CAD build for the part. Positions are in the model's coordinates, mm. Face numbers are marked on the shaded views. A direction names the side the tool comes from. Give positions to 0.01 mm unless a question says otherwise; leave off trailing zeros. Write each loop counter-clockwise with the first axis right and the second up, starting at its lowest first coordinate (ties: lowest second). Pieces come first, ordered by that corner, then holes. Notation, with made-up numbers: (14, 62.5) - (44, 62.5) arc R11 cw to (44, 69.5) - close; hole circle Ø4 at (-14, 12). An arc over 180 degrees is marked (long way). Put each result on its own line as item: value. Start each with the question number.
1. Cut at C-C on y = 10.25. List the corners of the cut face in (x, z).
2. Wall check: line 1 (X direction, y = 7.25, z = 0); line 2 (Z direction, x = 1, y = 11.5); line 3 (Z direction, x = -5.75, y = -1.5). Give the ranges that are in metal, low to high.
3. Cut at B-B on y = -0.5. List the corners of the cut face in (x, z).
4. Tool access for the marked faces 1, 2 and 3: list every direction of +Z, -Z, +X, -X, +Y, -Y with a clear straight run to the whole face (end or side of a thin tool).
5. Drop flat-ended pins along their axis: pin 1 (5 mm diameter, centred on x = 7, y = -3, fed in from +Z); pin 2 (3 mm diameter, centred on y = -0.5, z = -7.5, fed in from +X); pin 3 (1.5 mm diameter, centred on x = -3.5, y = -2.5, fed in from -Z); pin 4 (5 mm diameter, centred on x = 4.5, z = -6, fed in from +Y). Give the stop position or say it passes through.
6. Mould opens along Z. For the marked faces 4, 5 and 6 say: +Z half, -Z half, draft (parallel to the pull), parting line (faces both ways), or undercut.
7. Cut at A-A on y = 6. List the corners of the cut face in (x, z).
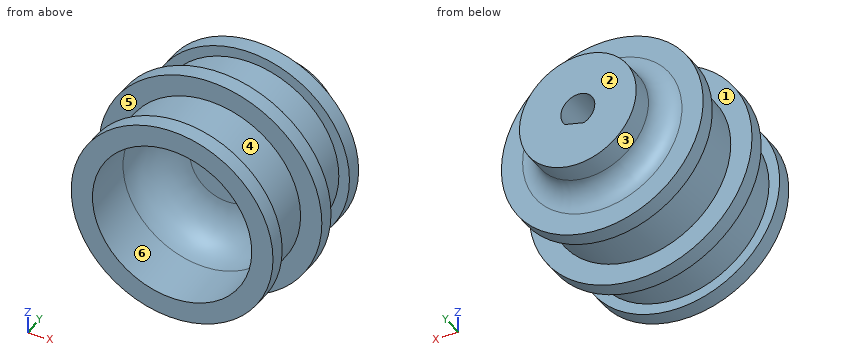
from build123d import *

# Parameters (mm, degrees)
ZAOKR_GLENIE1_R            = 2
WYTNIJ_WYCI_GNI_CIE1_DEPTH = 19


with BuildPart() as part:
    # Szkic1 → Obrót1 (revolve)
    with BuildSketch(Plane.XY):
        with BuildLine():
            Line((7.5, -4.799176992), (7.5, 0.200823008))
            ThreePointArc((7.5, 0.200823008), (6.328427125, 3.029250132), (3.5, 4.200823008))
            Line((3.5, 4.200823008), (0, 4.200823008))
            Line((0, 4.200823008), (0, 13.200823008))
            Line((0, 13.200823008), (5.5, 13.200823008))
            Line((5.5, 13.200823008), (5.5, 9.200823008))
            Line((5.5, 9.200823008), (9.5, 9.200823008))
            Line((9.5, 9.200823008), (9.5, 7.700823008))
            Line((9.5, 7.700823008), (8.5, 7.700823008))
            Line((8.5, 7.700823008), (8.5, 2.950823008))
            Line((8.5, 2.950823008), (10.5, 2.950823008))
            Line((10.5, 2.950823008), (10.5, 1.450823008))
            Line((10.5, 1.450823008), (8.5, 1.450823008))
            Line((8.5, 1.450823008), (8.5, -3.299176992))
            Line((8.5, -3.299176992), (9.5, -3.299176992))
            Line((9.5, -3.299176992), (9.5, -4.799176992))
            Line((9.5, -4.799176992), (7.5, -4.799176992))
        make_face()
    revolve(axis=Axis((0, -15.783107462, 0), (0, 1, 0)))

    # Zaokrąglenie1
    zaokr_glenie1_edges = [part.edges().sort_by_distance(p)[0] for p in [
        (-5.5, 9.200823008, 0),
    ]]
    fillet(zaokr_glenie1_edges, radius=ZAOKR_GLENIE1_R)

    # Szkic2 → Wytnij-wyciągnięcie1 (cut, through all)
    with BuildSketch(Plane(origin=(0, 13.200823008, 0), x_dir=(1, 0, 0), z_dir=(0, 1, 0))):
        with BuildLine():
            Line((-0.568761348, 1.49549675), (1.234520551, 1.017820716))
            ThreePointArc((1.234520551, 1.017820716), (-0.409697971, -1.546656902), (-0.568761348, 1.49549675))
        make_face()
    extrude(amount=-WYTNIJ_WYCI_GNI_CIE1_DEPTH, mode=Mode.SUBTRACT)


solid = part.part
Report:
1. outline: circle Ø11.48 at (0, 0); hole (-0.57, -1.5) - (1.23, -1.02) arc R1.6 ccw (long way) to start
2. line 1: x = -8.5 to -1.6, 1.6 to 8.5
2. line 2: z = -5.41 to -1.08, 1.25 to 5.41
2. line 3: z = -6.26 to -4.82, 4.82 to 6.26
3. outline: circle Ø17 at (0, 0); hole circle Ø15 at (0, 0)
4. face 1: none
4. face 2: +Z, -Z, +X, -X, +Y
4. face 3: +Y
5. pin 1: stops at z = 8.36
5. pin 2: stops at x = 6.02
5. pin 3: stops at z = -8.04
5. pin 4: stops at y = 13.2
6. face 4: parting line
6. face 5: draft
6. face 6: undercut
7. outline: circle Ø17 at (0, 0); hole (-0.57, -1.5) - (1.23, -1.02) arc R1.6 ccw (long way) to start
